Geometry: final body of the model. Coordinates: model frame, mm. A direction names the side the tool comes from. Give positions to 0.01 mm unless a question says otherwise; leave off trailing zeros. Loops run counter-clockwise (first coordinate to the right, second up) from the corner with the lowest first, then second, coordinate; pieces in that order, holes last. Notation, with made-up numbers: (-38.75, -33.5) -> (-19.75, -33.5) arc R25 ccw to (-19.75, 3.5) -> close; hole circle Ø9 at (59.5, 84.5). An arc over 180 degrees is marked (long way). One line per question, with ' | ' between items. Start each with the question number.
Item 1: Set-up query: faces 5 (the flat face through (43.5, 2, -2)), 6 (the flat face through (-47, 2, 0)), 7 (the flat face through (-44, 0, -6)), 8 (the flat face through (-34.75, 0, -1)), 9 (the flat face through (-27.9, -8, -2)). Return all of +Z, -Z, +X, -X, +Y, -Y with unobstructed straight access to the full face (end or side cutting, diameter ignored); none if empty.
Item 2: Section C-C on x = -10. Return loops of the section in (y, z), then the cut area to 3 significant figures.
Item 3: Section B-B on y = -4. Return loops of the section in (x, z), then the cut area to 3 significant figures.
Item 4: Material intervals for line 1 along X through (y, z) = (2.5, -0.25); line 2 along Y through (x, z) = (3, -2.5); line 3 along X through (y, z) = (-3.75, -0.5), sorted ascending. Write a range as [from, to].
Item 5: Section A-A on x = 10.5. Return loops of the section in (y, z), then the cut area to 3 significant figures.
Item 6: Pin query (flat end, axial travel): P1, Ø0.6, axis at y = 0, z = -2, coming from the +X side; P2, Ø1.6, axis at x = -11.5, y = -8, coming from the -Z side; P3, Ø0.6, axis at y = 8, z = -0.5, coming from the -X side. Return the tip coordinate at first contact, or that it passes through.
Item 7: Mould query, pull axis Y, two halves, no side actions, for faces 1 (the flat face through (-51, -2, -4)), 2 (the flat face through (47, -5, -2)), 3 (the flat face through (-1.6, -0.03, -4.06)), 4 (the flat face through (-34, 7, -3)). Classes: released by +Y, released by -Y, zero draft, split by the parting line, or undercut.
from build123d import *

# Parameters (mm, degrees)
SKETCH1_W            = 102
SKETCH1_H            = 18
BOSS_EXTRUDE1_DEPTH  = 2
BOSS_EXTRUDE2_DEPTH  = 18
SKETCH4_W            = 81
SKETCH4_H            = 2
BOSS_EXTRUDE3_DEPTH  = 6
SKETCH5_W            = 2.3
SKETCH5_H            = 2
SKETCH5_W_2          = 1.7
CUT_EXTRUDE1_DEPTH   = 6
SKETCH6_W            = 1.7
SKETCH6_H            = 2
BOSS_EXTRUDE4_DEPTH  = 4
CUT_EXTRUDE2_DEPTH   = 20
SKETCH8_W            = 2
SKETCH8_H            = 6
BOSS_EXTRUDE5_DEPTH  = 1
SKETCH10_W           = 3.5
SKETCH10_H           = 6
BOSS_EXTRUDE6_DEPTH  = 1
SKETCH11_W           = 1.5
SKETCH11_H           = 6
BOSS_EXTRUDE7_DEPTH  = 8
BOSS_EXTRUDE8_DEPTH  = 6
RIB1_REACH           = 54.402
SKETCH17_WALL_W      = 117.434725866
SKETCH17_WALL_H      = 4
CHAMFER1_SIZE        = 0.5
SKETCH18_W           = 7.5
SKETCH18_H           = 3.05
BOSS_EXTRUDE10_DEPTH = 4
SKETCH19_W           = 26.1754507
SKETCH19_H           = 11
CUT_EXTRUDE3_DEPTH   = 1
SKETCH20_W           = 2.3
SKETCH20_H           = 1
CUT_EXTRUDE4_DEPTH   = 21


with BuildPart() as part:
    # Sketch1 → Boss-Extrude1 (new body)
    with BuildSketch(Plane.XY):
        Rectangle(SKETCH1_W, SKETCH1_H)
    extrude(amount=BOSS_EXTRUDE1_DEPTH)

    # Sketch2 → Boss-Extrude2 (add)
    with BuildSketch(Plane(origin=(0, 9, 0), x_dir=(1, 0, 0), z_dir=(0, 1, 0))):
        Polygon((-43.5, 0), (-40.5, 0), (-40.5, 6), (-51, 6), (-51, 3.05), (-43.5, 3.05), align=None)
        Polygon((40.5, 6), (40.5, 0), (43.5, 0), (43.5, 3.05), (51, 3.05), (51, 6), align=None)
    extrude(amount=-BOSS_EXTRUDE2_DEPTH)

    # Sketch4 → Boss-Extrude3 (add)
    with BuildSketch(Plane(origin=(0, 0, 0), x_dir=(-1, 0, 0), z_dir=(0, 0, -1))):
        with Locations((0, 8)):
            Rectangle(SKETCH4_W, SKETCH4_H)
        with Locations((0, -8)):
            Rectangle(SKETCH4_W, SKETCH4_H)
    extrude(amount=BOSS_EXTRUDE3_DEPTH)

    # Sketch5 → Cut-Extrude1 (cut)
    with BuildSketch(Plane(origin=(0, 0, -6), x_dir=(-1, 0, 0), z_dir=(0, 0, -1))):
        with Locations((26.75, -8)):
            Rectangle(SKETCH5_W, SKETCH5_H)
        with Locations((26.75, 8)):
            Rectangle(SKETCH5_W, SKETCH5_H)
        with Locations((-20.25, 8)):
            Rectangle(SKETCH5_W_2, SKETCH5_H)
        with Locations((-20.25, -8)):
            Rectangle(SKETCH5_W_2, SKETCH5_H)
    extrude(amount=-CUT_EXTRUDE1_DEPTH, mode=Mode.SUBTRACT)

    # Sketch6 → Boss-Extrude4 (add)
    with BuildSketch(Plane(origin=(0, 0, -6), x_dir=(-1, 0, 0), z_dir=(0, 0, -1))):
        with Locations((-20.25, 8)):
            Rectangle(SKETCH6_W, SKETCH6_H)
        with Locations((-20.25, -8)):
            Rectangle(SKETCH6_W, SKETCH6_H)
    extrude(amount=-BOSS_EXTRUDE4_DEPTH)

    # Sketch7 → Cut-Extrude2 (cut)
    with BuildSketch(Plane(origin=(0, 9, 0), x_dir=(1, 0, 0), z_dir=(0, 1, 0))):
        Polygon((18.810082021, 0), (12.361738872, 6), (14.563742638, 6), (19.4, 1.5), (20.041328573, 1.5), (20.041328573, 0), align=None)
    extrude(amount=-CUT_EXTRUDE2_DEPTH, mode=Mode.SUBTRACT)

    # Sketch8 → Boss-Extrude5 (add)
    with BuildSketch(Plane(origin=(0, 0, 0), x_dir=(-1, 0, 0), z_dir=(0, 0, -1))):
        with Locations((33.75, 0)):
            Rectangle(SKETCH8_W, SKETCH8_H)
    extrude(amount=BOSS_EXTRUDE5_DEPTH)

    # Sketch10 → Boss-Extrude6 (add)
    with BuildSketch(Plane(origin=(0, 0, -1), x_dir=(-1, 0, 0), z_dir=(0, 0, -1))):
        with Locations((33, 0)):
            Rectangle(SKETCH10_W, SKETCH10_H)
    extrude(amount=BOSS_EXTRUDE6_DEPTH)

    # Sketch11 → Boss-Extrude7 (add)
    with BuildSketch(Plane(origin=(0, 0, 0), x_dir=(-1, 0, 0), z_dir=(0, 0, -1))):
        with Locations((5.8, 0)):
            Rectangle(SKETCH11_W, SKETCH11_H)
    extrude(amount=BOSS_EXTRUDE7_DEPTH)

    # Sketch12 → Boss-Extrude8 (add)
    with BuildSketch(Plane.XZ.offset(3)):
        Polygon((-6.55, -8), (-7.55, -6), (-6.55, -6), align=None)
    extrude(amount=-BOSS_EXTRUDE8_DEPTH)

    # Sketch17 wall → Rib1 (add, up to next)
    with BuildSketch(Plane(origin=(-1.55, 0, -4), x_dir=(0.658504607869, 0, 0.752576694707), z_dir=(0.752576694707, 0, -0.658504607869)), mode=Mode.PRIVATE) as rib1_sk1:
        Rectangle(SKETCH17_WALL_W, SKETCH17_WALL_H)
    rib1_tool1 = extrude(rib1_sk1.sketch, amount=-RIB1_REACH, mode=Mode.PRIVATE) - part.part
    add(rib1_tool1.solids().sort_by_distance((-1.55, 0, -4))[0])

    # Chamfer1
    chamfer1_edges = [part.edges().sort_by_distance(p)[0] for p in [
        (-31.25, 0, -1),
    ]]
    chamfer(chamfer1_edges, length=CHAMFER1_SIZE)

    # Sketch18 → Boss-Extrude10 (add)
    with BuildSketch(Plane.XZ.offset(9)):
        with Locations((47.25, -1.525)):
            Rectangle(SKETCH18_W, SKETCH18_H)
        with Locations((-47.25, -1.525)):
            Rectangle(SKETCH18_W, SKETCH18_H)
    extrude(amount=-BOSS_EXTRUDE10_DEPTH)

    # Sketch19 → Cut-Extrude3 (cut)
    with BuildSketch(Plane(origin=(0, 0, 0), x_dir=(-1, 0, 0), z_dir=(0, 0, -1))):
        with Locations((19.63772535, 0)):
            Rectangle(SKETCH19_W, SKETCH19_H)
    extrude(amount=-CUT_EXTRUDE3_DEPTH, mode=Mode.SUBTRACT)

    # Sketch20 → Cut-Extrude4 (cut)
    with BuildSketch(Plane(origin=(0, 9, 0), x_dir=(1, 0, 0), z_dir=(0, 1, 0))):
        with Locations((-26.75, -0.5)):
            Rectangle(SKETCH20_W, SKETCH20_H)
    extrude(amount=-CUT_EXTRUDE4_DEPTH, mode=Mode.SUBTRACT)


solid = part.part
Result sheet:
1) face 5: +X, +Y | face 6: -X, +Y | face 7: -Z, -X, +Y, -Y | face 8: -Z | face 9: -Z, +Y, -Y
2) outline: (-9, -6) -> (-7, -6) -> (-7, 0) -> (-5.5, 0) -> (-5.5, 1) -> (5.5, 1) -> (5.5, 0) -> (7, 0) -> (7, -6) -> (9, -6) -> (9, 2) -> (-9, 2) -> close | area: 49.0 mm²
3) outline: (-51, -6) -> (-40.5, -6) -> (-40.5, 0) -> (-32.73, 0) -> (-32.73, 1) -> (-6.55, 1) -> (-6.55, 0) -> (40.5, 0) -> (40.5, -6) -> (51, -6) -> (51, -3.05) -> (43.5, -3.05) -> (43.5, 0) -> (51, 0) -> (51, 2) -> (-51, 2) -> (-51, 0) -> (-43.5, 0) -> (-43.5, -3.05) -> (-51, -3.05) -> close | area: 258 mm²
4) line 1: x = [-43.5, -40.5], [-34.75, -32.75], [-6.55, -5.05], [40.5, 43.5] | line 2: y = [-9, -7], [7, 9] | line 3: x = [-43.5, -40.5], [40.5, 43.5]
5) outline: (-9, -6) -> (-7, -6) -> (-7, 0) -> (7, 0) -> (7, -6) -> (9, -6) -> (9, 2) -> (-9, 2) -> close | area: 60.0 mm²
6) P1: stops at x = 43.5 | P2: stops at z = -6 | P3: stops at x = -43.5
7) face 1: zero draft | face 2: released by +Y | face 3: undercut | face 4: undercut
